Print and shaded views of the part. All mm, measured from the part's lowest x, y and z. A direction names the side the tool comes from. Give positions to 0.01 mm unless a question says otherwise; leave off trailing zeros. Write each loop counter-clockwise with the first axis right and the second up, starting at its lowest first coordinate (ties: lowest second). Pieces come first, ordered by that corner, then holes.
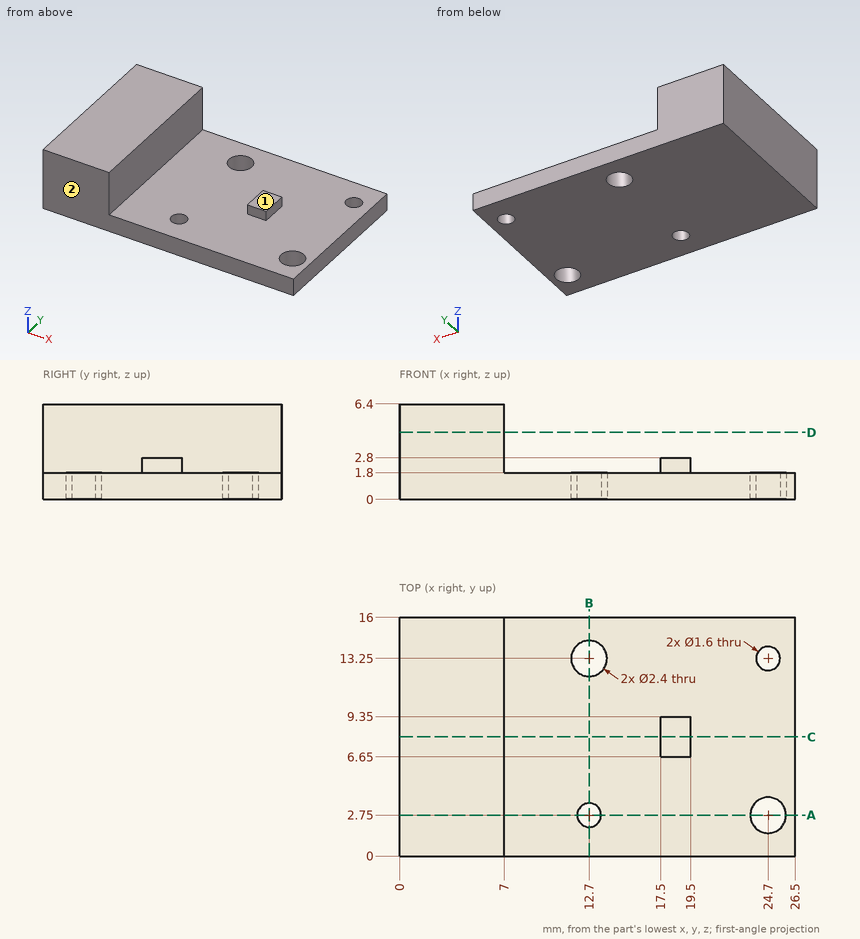
1. Saw through at D-D on z = 4.5. Give the cut face in (x, y), plus the area to 3 significant figures.
2. Saw through at C-C on y = 8. Give the cut face in (x, z).
3. 3-axis set-ups, long thin cutter, end or side, ignore diameter. For the marked faces 1 and 2: which of +Z, -Z, +X, -X, +Y, -Y reach the whole face in a straight line?
4. Drill centre lines: line 1 along Y through (x, z) = (12.7, 0.9); line 2 along Y through (x, z) = (24.7, 0.8); line 3 along X through (y, z) = (9, 2.75). Where is each one in solid material? Low to high.
5. Saw through at B-B on x = 12.7. Give the cut face in (y, z), plus the area to 3 significant figures.
6. Drop flat-ended pins along their axis: pin 1 (6 mm diameter, centred on x = 17, y = 10, fed in from +Z); pin 2 (5 mm diameter, centred on x = 13.5, y = 8, fed in from +Z); pin 3 (1.4 mm diameter, centred on y = 9, z = 4.5, fed in from +X). Give the stop position or say it passes through.
7. Saw through at A-A on y = 2.75. Give the cut face in (x, z).
Outcome:
1. outline: (0, 0) - (7, 0) - (7, 16) - (0, 16) - close
1. area: 112 mm2
2. outline: (0, 0) - (26.5, 0) - (26.5, 1.8) - (19.5, 1.8) - (19.5, 2.8) - (17.5, 2.8) - (17.5, 1.8) - (7, 1.8) - (7, 6.4) - (0, 6.4) - close
3. face 1: +Z, +X, +Y, -Y
3. face 2: +Z, -Z, +X, -X, -Y
4. line 1: y = 0 to 1.95, 3.55 to 12.05, 14.45 to 16
4. line 2: y = 0 to 1.55, 3.95 to 12.45, 14.05 to 16
4. line 3: x = 0 to 7, 17.5 to 19.5
5. outline: (0, 0) - (1.95, 0) - (1.95, 1.8) - (0, 1.8) - close; (3.55, 0) - (12.05, 0) - (12.05, 1.8) - (3.55, 1.8) - close; (14.45, 0) - (16, 0) - (16, 1.8) - (14.45, 1.8) - close
5. area: 21.6 mm2
6. pin 1: stops at z = 2.8
6. pin 2: stops at z = 1.8
6. pin 3: stops at x = 7
7. outline: (0, 0) - (11.9, 0) - (11.9, 1.8) - (7, 1.8) - (7, 6.4) - (0, 6.4) - close; (13.5, 0) - (23.5, 0) - (23.5, 1.8) - (13.5, 1.8) - close; (25.9, 0) - (26.5, 0) - (26.5, 1.8) - (25.9, 1.8) - close
